Answer from the drawing. Dimensions are ordinates in mm from the lowest x, y and z of the part. Round coordinates to 2 decimals unless told otherwise and drop trailing zeros. Write each loop counter-clockwise with the first axis right and the second up, starting at its lowest first coordinate (ties: lowest second). Pieces come first, ordered by that corner, then holes. Notation, with made-up numbers: M 14.5,69 L 28.5,69 A14 cw 28.5,95 Z; hole C 17.25,-36.5 d6. An arc over 180 degrees is marked long. One line per item, written item: value. Start each with the question number.
(1) Given P1, Ø3, axis at x = 6.5, y = 7.5, coming from the -Z side; P2, Ø4, axis at x = 5, y = 10, coming from the +Z side; P3, Ø6, axis at x = 20.5, y = 3, coming from the +Z side, each flat-ended and moving along its own axis, determine where each tip first touches the part or whether it passes through.
(2) Section A-A (z = 3.5) is taken. Determine the outline of the cut face in (x, y) (3 decimals), plus the area to 3 significant figures.
(3) Section B-B (y = 3.5) is taken. Determine the outline of the cut face in (x, z).
(4) Section C-C (x = 9) is taken. Determine the outline of the cut face in (y, z) (3 decimals), plus the area to 3 significant figures.
(5) Consider probe 1 along Z at (x, y) = (29.5, 5.25); probe 2 along X at (y, z) = (8.75, 2); probe 3 along Z at (x, y) = (21.5, 13.5). Determine where each line is inside the solid, lowest interval first.
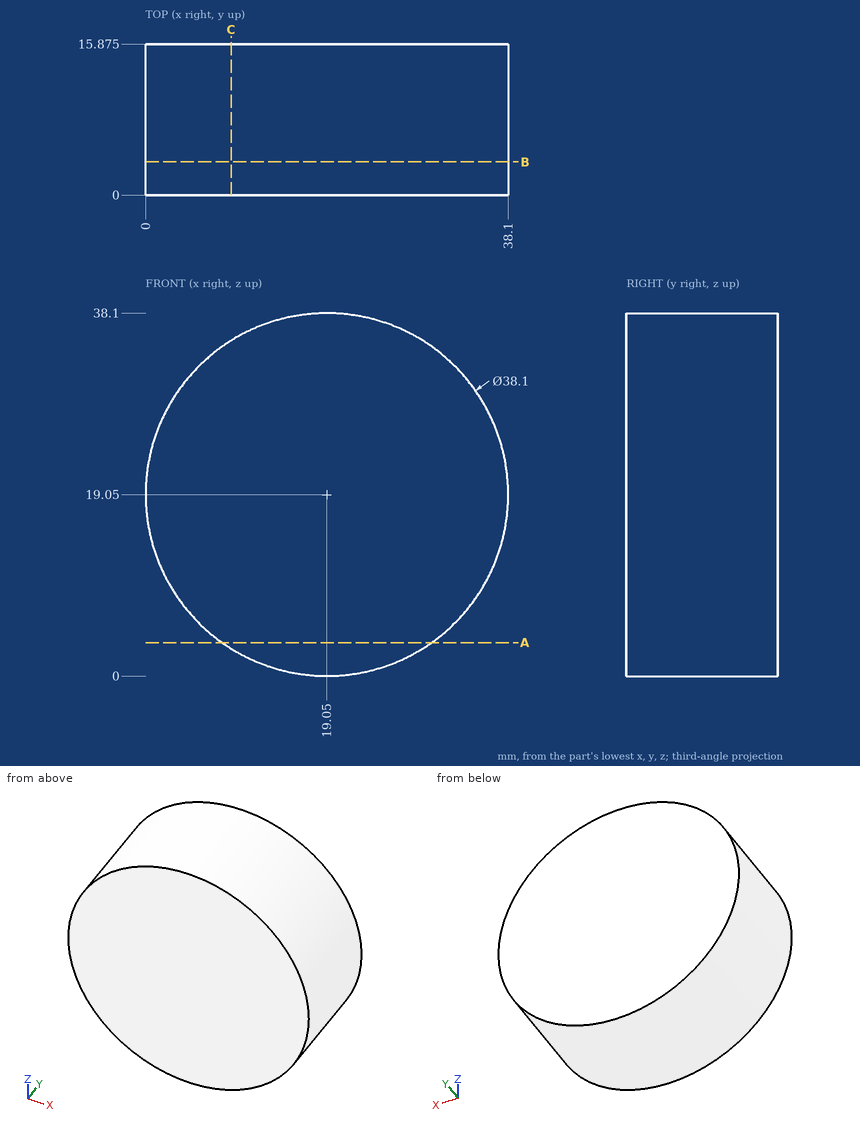
Recorded:
1. P1: stops at z = 3.53
1. P2: stops at z = 33.8
1. P3: stops at z = 38.1
2. outline: M 8.045,0 L 30.055,0 L 30.055,15.875 L 8.045,15.875 Z
2. area: 349 mm2
3. outline: C 19.05,19.05 d38.1
4. outline: M 0,2.867 L 15.875,2.867 L 15.875,35.233 L 0,35.233 Z
4. area: 514 mm2
5. probe 1: z = 3.12 to 34.98
5. probe 2: x = 10.55 to 27.55
5. probe 3: z = 0.16 to 37.94
